Verification items for the finished model (mm, model axes). Round coordinates to 2 decimals unless told otherwise and drop trailing zeros. Order: outer loops, then holes, each group sorted by start corner. A loop starts at its lowest first (then second) coordinate and runs counter-clockwise, first axis right, second up. Notation, with made-up numbers: (85, -34) -> (127, -34) arc R5 cw to (127, -26) -> close; hole circle Ø10 at (79, 7.25). An arc over 180 degrees is marked (long way). Return JSON: item names as keys, results as strings. Group by question number.
Item 1: Sectioned sample at B-B on z = 0.75. Record the cut outline in (x, y).
Item 2: Sectioned sample at C-C on y = 12.5. Record the cut outline in (x, z), plus the area to 3 significant figures.
Item 3: Draft check along X on faces 1 (the flat face through (-5.2, 6, 0)), 2 (the flat face through (0, 3, 5)), 3 (the flat face through (0, 6, 3.95)). Enter one of: pulls with the +X half, pulls with the -X half, needs draft (parallel to the pull), parting line crosses it, or undercut.
Item 4: Sectioned sample at D-D on z = -8.5. Record the cut outline in (x, y), plus the area to 3 significant figures.
Item 5: Depth check by flat-ended pin: pin 1 Ø2 at (x, y) = (0.5, 5.5) entering from +Z; pin 2 Ø2 at (x, y) = (1, 6) entering from -Z; pin 3 Ø12 at (x, y) = (0.5, 21.5) entering from -Z. Enter the tip coordinate at first touch or a pass-through.
Item 6: Sectioned sample at A-A on x = -0.75. Record the cut outline in (y, z).
Item 7: Scan lines: probe 1 along Z at (x, y) = (-1.25, 9.5); probe 2 along X at (y, z) = (5.75, 0.75); probe 3 along X at (y, z) = (14.25, 4.5). Record each from-to range of solid material in increasing order. Write a range as from..to.
```python
from build123d import *

# Parameters (mm, degrees)
ESQUISSE3_W             = 10.4
ESQUISSE3_H             = 7.9
ESQUISSE3_W_2           = 10
ESQUISSE3_H_2           = 7.5
ENL_V_MAT_EXTRU_1_DEPTH = 10
ESQUISSE5_W             = 20
ESQUISSE5_H             = 20
ENL_V_MAT_EXTRU_2_DEPTH = 3


with BuildPart() as part:
    # Esquisse2 → Révolution1 (revolve)
    with BuildSketch(Plane(origin=(0, 0, 0), x_dir=(0, 0, -1), z_dir=(1, 0, 0))):
        with BuildLine():
            Line((0, 0), (0, 25))
            ThreePointArc((0, 25), (12.5, 12.5), (0, 0))
        make_face()
    revolve(axis=Axis((0, 0, 0), (0, 1, 0)))

    # Esquisse3 → Enlèv. mat.-Extru.1 (cut)
    # profile 1 of 2: a face of its own
    with BuildSketch(Plane(origin=(0, 0, 0), x_dir=(1, 0, 0), z_dir=(0, 1, 0))):
        Rectangle(ESQUISSE3_W, ESQUISSE3_H)
        Rectangle(ESQUISSE3_W_2, ESQUISSE3_H_2, mode=Mode.SUBTRACT)
    # profile 2 of 2: a face of its own
    with BuildSketch(Plane(origin=(0, 0, 0), x_dir=(1, 0, 0), z_dir=(0, 1, 0))):
        Rectangle(ESQUISSE3_W_2, ESQUISSE3_H_2)
    extrude(amount=ENL_V_MAT_EXTRU_1_DEPTH, mode=Mode.SUBTRACT)

    # Esquisse5 → Enlèv. mat.-Extru.2 (cut)
    with BuildSketch(Plane(origin=(0, 0, 0), x_dir=(1, 0, 0), z_dir=(0, 1, 0))):
        Rectangle(ESQUISSE5_W, ESQUISSE5_H)
    extrude(amount=ENL_V_MAT_EXTRU_2_DEPTH, mode=Mode.SUBTRACT)


solid = part.part
```
Recorded:
{
 "1": {"outline": "(-8.09, 3) -> (-5.2, 3) -> (-5.2, 10) -> (5.2, 10) -> (5.2, 3) -> (8.09, 3) arc R12.48 ccw (long way) to start"},
 "2": {"outline": "circle Ø25 at (0, 0)", "area": "491 mm²"},
 "3": {"face 1": "undercut", "face 2": "needs draft", "face 3": "undercut"},
 "4": {"outline": "circle Ø18.33 at (0, 12.5)", "area": "264 mm²"},
 "5": {"pin 1": "z = 10.96", "pin 2": "z = -11.19", "pin 3": "z = -12.13"},
 "6": {"outline": "(3, -8.09) arc R12.48 ccw (long way) to (3, 8.09) -> (3, 3.95) -> (10, 3.95) -> (10, -3.95) -> (3, -3.95) -> close"},
 "7": {"probe 1": "-12.07..-3.95, 3.95..12.07", "probe 2": "-10.49..-5.2, 5.2..10.49", "probe 3": "-11.53..11.53"}
}
